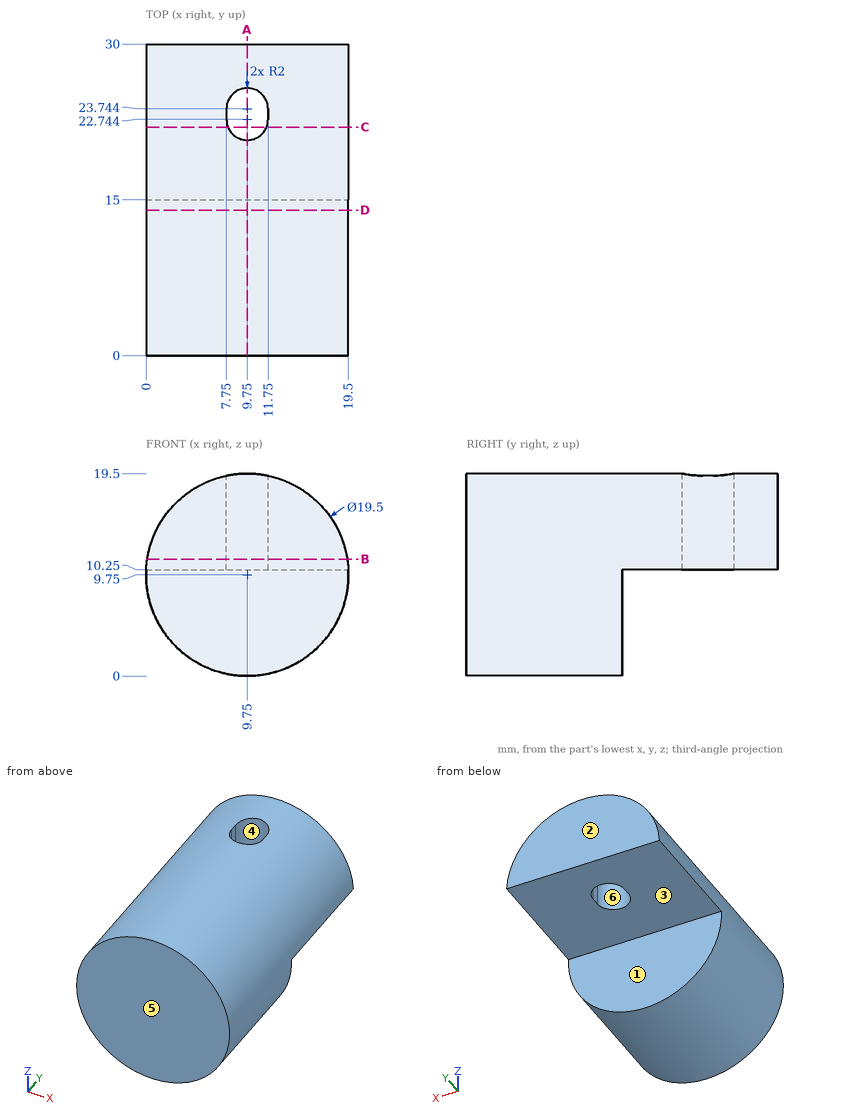
Could you check a few things on this drawing? It's one solid part, dimensions in mm from its lowest x, y, z. A direction names the side the tool comes from. Give positions to 0.01 mm unless a question says otherwise; leave off trailing zeros. Order: outer loops, then holes, each group sorted by start corner. A loop starts at its lowest first (then second) coordinate and runs counter-clockwise, first axis right, second up. Notation, with made-up numbers: (-6.75, -25.5) - (31.25, -25.5) arc R12 cw to (31.25, -7.5) - close; hole circle Ø1 at (17, 63.5). An arc over 180 degrees is marked (long way). Return JSON: item names as keys, results as strings. Group by question number.
Q1. Suppose I cut it at C-C, the plane y = 22. Please give me the cut outline in (x, z), and give its area (3 significant figures).
Q2. Which directions (+Z, -Z, +X, -X, +Y, -Y) give clear straight access to the entire face, cutting with the end or side of a thin tool? Please do the marked faces 1 and 2.
Q3. Thinking about a two-plate mould opening in Y: for the marked faces 3, 4, 5 and 6, which applies, pulls with the +Y half, pulls with the -Y half, needs draft (parallel to the pull), parting line crosses it, or undercut?
Q4. Suppose I cut it at D-D, the plane y = 14. Please give me the cut outline in (x, z).
Q5. Please list where these lines run through material, in increasing order: line 1 along Y through (x, z) = (3.5, 6); line 2 along Y through (x, z) = (11.25, 16.75); line 3 along Y through (x, z) = (9, 14.5). Write a range as [from, to].
Q6. Will these pins go through, and if not, where does the flat tip stop? pin 1 Ø5 at (y, z) = (24.5, 12) entering from -X; pin 2 Ø8 at (x, y) = (6, 23) entering from -Z; pin 3 Ø5 at (x, z) = (7, 6) entering from +Y.
Q7. Suppose I cut it at A-A, the plane x = 9.75. Please give me the cut outline in (y, z).
Q8. Suppose I cut it at B-B, the plane z = 11.25. Please give me the cut outline in (x, y).
Resolved:
{
 "1": {"outline": "(0.01, 10.25) - (7.89, 10.25) - (7.89, 19.32) arc R9.75 ccw to start; (11.61, 10.25) - (19.49, 10.25) arc R9.75 ccw to (11.61, 19.32) - close", "area": "105 mm2"},
 "2": {"face 1": "-Z, +X, -X, +Y", "face 2": "+Z, -Z, +X, -X, +Y"},
 "3": {"face 3": "needs draft", "face 4": "undercut", "face 5": "pulls with the -Y half", "face 6": "undercut"},
 "4": {"outline": "circle Ø19.5 at (9.75, 9.75)"},
 "5": {"line 1": "y = [0, 15]", "line 2": "y = [0, 21.42], [25.07, 30]", "line 3": "y = [0, 20.89], [25.6, 30]"},
 "6": {"pin 1": "stops at x = 0.01", "pin 2": "stops at z = 10.25", "pin 3": "stops at y = 15"},
 "7": {"outline": "(0, 0) - (15, 0) - (15, 10.25) - (20.74, 10.25) - (20.74, 19.5) - (0, 19.5) - close; (25.74, 10.25) - (30, 10.25) - (30, 19.5) - (25.74, 19.5) - close"},
 "8": {"outline": "(0.12, 0) - (19.38, 0) - (19.38, 30) - (0.12, 30) - close; hole (7.75, 22.74) arc R2 ccw to (11.75, 22.74) - (11.75, 23.74) arc R2 ccw to (7.75, 23.74) - close"}
}
